Check sheet for the modelled part. Datum: model origin and axes. Units: mm. A direction names the side the tool comes from. Coordinates: 2 decimals unless noted, no trailing zeros. Write each loop counter-clockwise with the first axis right and the second up, starting at its lowest first coordinate (ties: lowest second). Pieces come first, ordered by that corner, then holes. Notation, with made-up numbers: M 49.25,78 L 74.25,78 A12 ccw 74.25,86 Z; hole C -11,-13.5 d3. An arc over 180 degrees is marked long. Answer as CSV lines item,"result". Start each with the question number.
Q1. Sectioned sample at A-A, the plane x = 0. Record the cut outline in (y, z) (3 decimals).
Q2. Mould release check, pull along Z, two halves, no side actions. Record for faces 1 (the cylindrical face through (-4.356, 4.785, -26.164)), 2 (the flat face through (15, 3, 31.75)), 3 (the flat face through (0, 6.35, 23)): pulls with the +Z half, pulls with the -Z half, needs draft (parallel to the pull), parting line crosses it, or undercut.
Q3. Sectioned sample at D-D, the plane x = -29.5. Record the cut outline in (y, z) (3 decimals).
Q4. Sectioned sample at B-B, the plane z = 0. Record the cut outline in (x, y) (3 decimals).
Q5. Sectioned sample at C-C, the plane z = -30.48. Record the cut outline in (x, y) (3 decimals), then the cut area to 3 significant figures.
Q6. Thickness scan on line 1 along X through (y, z) = (2, 0) (3 decimals); line 2 along Y through (x, z) = (-35, 1.5) (3 decimals); line 3 along Z through (x, y) = (15.24, 4.5). Record the ranges inside material, lowest first. Write a range as from..to.
Q7. Access from +Z, -Z, +X, -X, +Y, -Y to the whole of each face (thin tool, end or side, straight path). Record for faces 4 (the cylindrical face through (38.857, 4.74, 11.068)), 5 (the flat face through (20.32, 3, 29)), 6 (the flat face through (15.875, 2, -23)), 7 (the flat face through (0, 3, 25.4)).
Q8. Depth check by flat-ended pin: pin 1 Ø1 at (x, y) = (11, 1.5) entering from -Z; pin 2 Ø3 at (y, z) = (1.5, 30) entering from -X; pin 3 Ø5 at (x, z) = (20, -13.5) entering from +Y (3 decimals). Enter the tip coordinate at first touch or a pass-through.
from build123d import *

# Parameters (mm, degrees)
SKETCH1_R                    = 3.175
SKETCH1_R_2                  = 1.5875
BOSS_EXTRUDE1_DEPTH          = 3.175
CUT_EXTRUDE1_REACH           = 61.599
BOSS_EXTRUDE2_DEPTH          = 3.175
TAP_DRILL_FOR_10_HELICOIL2_D = 5.1054
FILLET1_R                    = 2.54
CUT_EXTRUDE2_REACH           = 61.146
SKETCH20_W                   = 20.32
SKETCH20_H                   = 6.35


with BuildPart() as part:
    # Sketch1 → Boss-Extrude1 (new body)
    with BuildSketch(Plane(origin=(0, 0, 0), x_dir=(1, 0, 0), z_dir=(0, 1, 0))):
        with BuildLine():
            Line((-20.32, 25.4), (-15.875, 25.4))
            Line((-15.875, 25.4), (0, 38.1))
            Line((0, 38.1), (15.875, 25.4))
            Line((15.875, 25.4), (20.32, 25.4))
            ThreePointArc((20.32, 25.4), (45.72, 0), (20.32, -25.4))
            Line((20.32, -25.4), (20.32, -31.75))
            Line((20.32, -31.75), (-20.32, -31.75))
            Line((-20.32, -31.75), (-20.32, -25.4))
            ThreePointArc((-20.32, -25.4), (-45.72, 0), (-20.32, 25.4))
        make_face()
        with Locations(Location((20.32, 0, 0), (0, 0, 270))):
            Circle(SKETCH1_R, mode=Mode.SUBTRACT)
        with Locations(Location((7.62, 21.997045256, 0), (0, 0, 270))):
            Circle(SKETCH1_R_2, mode=Mode.SUBTRACT)
        with Locations(Location((-20.32, 0, 0), (0, 0, 270))):
            Circle(SKETCH1_R, mode=Mode.SUBTRACT)
        with Locations(Location((-7.62, 21.997045256, 0), (0, 0, 270))):
            Circle(SKETCH1_R_2, mode=Mode.SUBTRACT)
    extrude(amount=BOSS_EXTRUDE1_DEPTH)

    # Sketch7 → Cut-Extrude1 (cut, up to next)
    with BuildSketch(Plane(origin=(0, 3.175, 0), x_dir=(1, 0, 0), z_dir=(0, 1, 0)), mode=Mode.PRIVATE) as cut_extrude1_sk1:
        with BuildLine():
            Line((-42.317045256, 12.7), (-39.017488468, 10.795))
            ThreePointArc((-39.017488468, 10.795), (-31.115, 18.697488468), (-20.32, 21.59))
            Line((-20.32, 21.59), (-15.875, 21.59))
            Line((-15.875, 21.59), (-15.875, 25.008038208))
            ThreePointArc((-15.875, 25.008038208), (-18.088875897, 25.301819801), (-20.32, 25.4))
            ThreePointArc((-20.32, 25.4), (-33.02, 21.997045256), (-42.317045256, 12.7))
        make_face()
    cut_extrude1_tool1 = extrude(cut_extrude1_sk1.sketch, amount=-CUT_EXTRUDE1_REACH, mode=Mode.PRIVATE) & part.part
    # Sketch7 → Cut-Extrude1 (cut, up to next)
    with BuildSketch(Plane(origin=(0, 3.175, 0), x_dir=(1, 0, 0), z_dir=(0, 1, 0)), mode=Mode.PRIVATE) as cut_extrude1_sk2:
        with BuildLine():
            Line((-15.875, 25.4), (-20.32, 25.4))
            ThreePointArc((-20.32, 25.4), (-18.088875897, 25.301819801), (-15.875, 25.008038208))
            Line((-15.875, 25.008038208), (-15.875, 25.4))
        make_face()
    cut_extrude1_tool2 = extrude(cut_extrude1_sk2.sketch, amount=-CUT_EXTRUDE1_REACH, mode=Mode.PRIVATE) & part.part
    cut_extrude1_1 = cut_extrude1_tool1.solids().sort_by_distance((-29.568041, 3.175, -20.060943))[0]
    add(cut_extrude1_1, mode=Mode.SUBTRACT)
    cut_extrude1_2 = cut_extrude1_tool2.solids().sort_by_distance((-16.984528, 3.175, -25.282569))[0]
    add(cut_extrude1_2, mode=Mode.SUBTRACT)
    cut_extrude1 = cut_extrude1_1 + cut_extrude1_2  # Cut-Extrude1 as one shape, for the pattern or mirror that repeats it

    # Sketch9 → Boss-Extrude2 (add)
    with BuildSketch(Plane(origin=(0, 3.175, 0), x_dir=(1, 0, 0), z_dir=(0, 1, 0))):
        with BuildLine():
            Line((-39.017488468, 10.795), (-42.317045256, 12.7))
            ThreePointArc((-42.317045256, 12.7), (-42.317045256, -12.7), (-20.32, -25.4))
            Line((-20.32, -25.4), (-20.32, -31.75))
            Line((-20.32, -31.75), (-10.16, -31.75))
            Line((-10.16, -31.75), (-10.16, -25.4))
            Line((-10.16, -25.4), (0, -25.4))
            Line((0, -25.4), (0, -21.59))
            Line((0, -21.59), (-20.32, -21.59))
            ThreePointArc((-20.32, -21.59), (-39.017488468, -10.795), (-39.017488468, 10.795))
        make_face()
        Polygon((0, 38.1), (-5.08, 34.036), (-5.08, 25.4), (0, 25.4), align=None)
    boss_extrude2 = extrude(amount=BOSS_EXTRUDE2_DEPTH)

    # Mirror1: Cut-Extrude1, Boss-Extrude2 across plane
    add(cut_extrude1.mirror(Plane(origin=(0, 0, 0), x_dir=(0, 0, 1), z_dir=(1, 0, 0))), mode=Mode.SUBTRACT)
    add(boss_extrude2.mirror(Plane(origin=(0, 0, 0), x_dir=(0, 0, 1), z_dir=(1, 0, 0))))

    # Tap Drill for #10 Helicoil2 (through all)
    with Locations(Plane(origin=(0, 6.35, 0), x_dir=(1, 0, 0), z_dir=(0, 1, 0))):
        with Locations((-15.24, -26.67), (15.24, -26.67), (0, 30.48)):
            Hole(TAP_DRILL_FOR_10_HELICOIL2_D / 2)

    # Fillet1
    fillet1_edges = [part.edges().sort_by_distance(p)[0] for p in [
        (5.08, 4.7625, -25.4),
        (0, 3.175, -38.1),
        (-5.08, 4.7625, -25.4),
    ]]
    fillet(fillet1_edges, radius=FILLET1_R)

    # Sketch20 → Cut-Extrude2 (cut, up to next)
    with BuildSketch(Plane(origin=(0, 3.175, 0), x_dir=(1, 0, 0), z_dir=(0, 1, 0)), mode=Mode.PRIVATE) as cut_extrude2_sk1:
        with Locations((0, -28.575)):
            Rectangle(SKETCH20_W, SKETCH20_H)
    cut_extrude2_tool1 = extrude(cut_extrude2_sk1.sketch, amount=-CUT_EXTRUDE2_REACH, mode=Mode.PRIVATE) & part.part
    add(cut_extrude2_tool1.solids().sort_by_distance((0, 3.175, 28.575))[0], mode=Mode.SUBTRACT)


solid = part.part
Output:
1,outline,"M 0,-37.387 L 6.35,-37.387 L 6.35,-33.033 L 0,-33.033 Z; M 0,-27.927 L 6.35,-27.927 L 6.35,-25.4 L 3.175,-25.4 L 3.175,21.59 L 6.35,21.59 L 6.35,25.4 L 0,25.4 Z"
2,face 1,"undercut"
2,face 2,"pulls with the +Z half"
2,face 3,"needs draft"
3,outline,"M 0,-19.541 L 3.175,-19.541 L 3.175,19.541 L 6.35,19.541 L 6.35,23.683 L 0,23.683 Z"
4,outline,"M -45.72,0 L -23.495,0 L -23.495,3.175 L -41.91,3.175 L -41.91,6.35 L -45.72,6.35 Z; M -17.145,0 L 17.145,0 L 17.145,3.175 L -17.145,3.175 Z; M 23.495,0 L 45.72,0 L 45.72,6.35 L 41.91,6.35 L 41.91,3.175 L 23.495,3.175 Z"
5,outline,"M -9.525,0 L -2.553,0 L -2.553,6.35 L -5.08,6.35 L -5.08,3.175 L -9.525,3.175 Z; M 2.553,0 L 9.525,0 L 9.525,3.175 L 5.08,3.175 L 5.08,6.35 L 2.553,6.35 Z"
5,area,"60.3 mm^2"
6,line 1,"x = -45.72..-23.495, -17.145..17.145, 23.495..45.72"
6,line 2,"y = 0..3.175"
6,line 3,"z = 21.59..24.12, 29.22..31.75"
7,face 4,"+Y"
7,face 5,"+Z, +X, +Y, -Y"
7,face 6,"-Z, +X, +Y, -Y"
7,face 7,"+Z, +Y, -Y"
8,pin 1,"stops at z = -29.7"
8,pin 2,"stops at x = -20.32"
8,pin 3,"stops at y = 3.175"
